Model file for the job. Use its own axes, mm. Face numbers are marked on the shaded views. A direction names the side the tool comes from. Coordinates: 2 decimals unless noted, no trailing zeros. Loops run counter-clockwise (first coordinate to the right, second up) from the corner with the lowest first, then second, coordinate; pieces in that order, holes last.
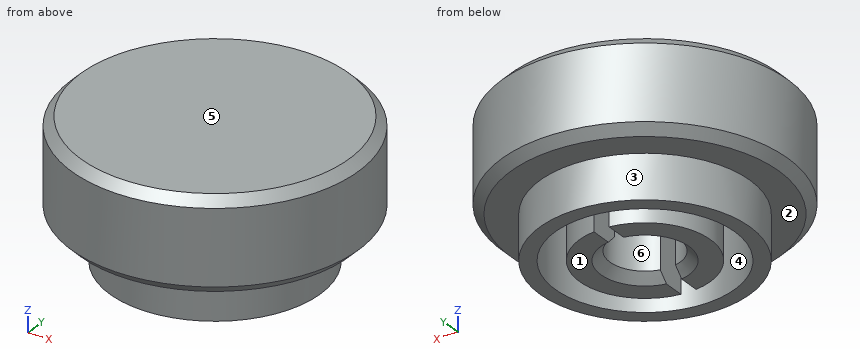
from build123d import *

# Parameters (mm, degrees)
SKETCH012_W     = 0.5
SKETCH012_H     = 5
POCKET002_DEPTH = 3
CHAMFER001_SIZE = 0.3


with BuildPart() as part:
    # Sketch011 → Revolution003 (revolve)
    with BuildSketch(Plane.XZ):
        Polygon((-3.45, 0), (-3.45, 1.452), (-4.699, 1.452), (-4.699, 4.5), (0, 4.5), (0, 3), (-1.15, 3), (-1.15, 0), (-2.15, 0), (-2.15, 3), (-2.95, 3), (-2.95, 0), align=None)
    revolve(axis=Axis((0, 0, 0), (0, 0, 1)))

    # Sketch012 → Pocket002 (cut)
    with BuildSketch(Plane.XY):
        Rectangle(SKETCH012_W, SKETCH012_H)
    extrude(amount=POCKET002_DEPTH, mode=Mode.SUBTRACT)

    # Chamfer001
    chamfer001_edges = [part.edges().sort_by_distance(p)[0] for p in [
        (4.699, 0, 4.5),
        (4.699, 0, 1.452),
        (1.15, 0, 0),
        (-0.897218, 0.719375, 0),
    ]]
    chamfer(chamfer001_edges, length=CHAMFER001_SIZE)


solid = part.part
Q1. Flat gauge pins, fed straight in: P1, Ø2, axis at x = 2, z = 3.5, coming from the +Y side; P2, Ø1, axis at y = 2, z = 2.5, coming from the +X side; P3, Ø0.8, axis at y = 1.5, z = 1.5, coming from the -X side. Where does each tip first touch, or does it go through?
Answers:
P1: stops at y = 4.59
P2: stops at x = 4.45
P3: stops at x = -4.55
Q2. Slice it at D-D (z = 3.7). List the corners of the cut face in (x, y).
Answers:
outline: circle Ø9.4 at (0, 0)
Q3. Slice it at A-A (z = 2.25). List the corners of the cut face in (x, y).
Answers:
outline: circle Ø9.4 at (0, 0); (-0.25, -2.14) - (-0.25, -1.12) arc R1.15 cw to (-0.25, 1.12) - (-0.25, 2.14) arc R2.15 ccw to start; (0.25, -2.14) arc R2.15 ccw to (0.25, 2.14) - (0.25, 1.12) arc R1.15 cw to (0.25, -1.12) - close; hole circle Ø5.9 at (0, 0)
Q4. Mould opens along Y. For the marked faces 3, 4, 5 and 6 say: +Y half, -Y half, draft (parallel to the pull), parting line (faces both ways), or undercut.
Answers:
face 3: parting line
face 4: undercut
face 5: draft
face 6: undercut
Q5. Slice it at C-C (x = 0). List the corners of the cut face in (y, z).
Answers:
outline: (-4.7, 1.75) - (-4.4, 1.45) - (-3.45, 1.45) - (-3.45, 0) - (-2.95, 0) - (-2.95, 3) - (2.95, 3) - (2.95, 0) - (3.45, 0) - (3.45, 1.45) - (4.4, 1.45) - (4.7, 1.75) - (4.7, 4.2) - (4.4, 4.5) - (-4.4, 4.5) - (-4.7, 4.2) - close
Q6. Drill centre lines: line 1 (X direction, y = 0, z = 0.75); line 2 (Y direction, x = -0.5, z = 2.6); line 3 (Y direction, x = 1.25, z = 2.9). Where is each one in solid material? Low to high.
Answers:
line 1: x = -3.45 to -2.95, -2.15 to -1.15, 1.15 to 2.15, 2.95 to 3.45
line 2: y = -4.67 to -2.91, -2.09 to -1.04, 1.04 to 2.09, 2.91 to 4.67
line 3: y = -4.53 to -2.67, -1.75 to 1.75, 2.67 to 4.53
Q7. Which spindle directions (+Z, -Z, +X, -X, +Y, -Y) get a long thin tool onto all of the face, cutting with end or side? Do the marked faces 1 and 2. Say none if no direction does.
Answers:
face 1: -Z, +X, -X, +Y, -Y
face 2: -Z
Q8. Slice it at B-B (y = 0). List the corners of the cut face in (x, z), and give its area (3 significant figures).
Answers:
outline: (-4.7, 1.75) - (-4.4, 1.45) - (-3.45, 1.45) - (-3.45, 0) - (-2.95, 0) - (-2.95, 3) - (-2.15, 3) - (-2.15, 0) - (-1.45, 0) - (-1.15, 0.3) - (-1.15, 3) - (1.15, 3) - (1.15, 0.3) - (1.45, 0) - (2.15, 0) - (2.15, 3) - (2.95, 3) - (2.95, 0) - (3.45, 0) - (3.45, 1.45) - (4.4, 1.45) - (4.7, 1.75) - (4.7, 4.2) - (4.4, 4.5) - (-4.4, 4.5) - (-4.7, 4.2) - close
area: 26.7 mm2
